Source: CAD feature listing. Evaluate the final solid. Frame: model axes, mm. Give positions to 0.01 mm unless a question says otherwise; leave off trailing zeros. Loops run counter-clockwise (first coordinate to the right, second up) from the corner with the lowest first, then second, coordinate; pieces in that order, holes last. Notation, with made-up numbers: M 80.5,-3.5 L 116.5,-3.5 A27 cw 116.5,31.5 Z; hole C 6.25,32 d10. An arc over 180 degrees is marked long. Put each result on its own line as item: value.
from build123d import *

# Parameters (mm, degrees)
F0_R     = 14.75
F1_DEPTH = 77
F2_R     = 9.55
F3_DEPTH = 77.001
F4_R     = 3


# Not quite as in the source:
# - a fillet or chamfer that OpenCascade refuses, or shapes differently, is made with other operations: its cross-section is extruded or revolved along the edge and cut away or added


with BuildPart() as f1:
    # F0 (on Top) → F1 (new body)
    with BuildSketch(Plane.XY):
        Circle(F0_R)
    extrude(amount=F1_DEPTH)

    # F2 (on Top) → F3 (cut, through all)
    with BuildSketch(Plane.XY):
        Circle(F2_R)
    extrude(amount=F3_DEPTH, mode=Mode.SUBTRACT)

    # F4
    f4_edges = [f1.edges().sort_by_distance(p)[0] for p in [
        (-14.75, 0, 77),
    ]]
    fillet(f4_edges, radius=F4_R)

    # F5: chamfer of 3 on 1 edges, made by hand

    # F5_s1 → F5_t2 (revolve, cut)
    with BuildSketch(Plane.XZ):
        Polygon((12.55, 77), (9.55, 74), (9.55, 77), align=None)
    revolve(axis=Axis((0, 0, 77), (0, 0, -1)), mode=Mode.SUBTRACT)


solid = f1.part
1. Contact query for flat-ended pins moving along their axis: P1, Ø2, axis at y = 1.5, z = 10.5, coming from the +X side; P2, Ø8, axis at y = 7, z = 19.5, coming from the -X side; P3, Ø3, axis at y = -6, z = 49.5, coming from the +X side. Output: stop coordinate, or through.
Found:
P1: x = 14.74
P2: x = -14.44
P3: x = 14.05
2. Section query A-A (x = 0). Output: boundary loops of the cut face in (y, z).
Found:
outline: M -14.75,0 L -9.55,0 L -9.55,74 L -12.46,76.91 A3 ccw -14.75,74 Z; M 9.55,0 L 14.75,0 L 14.75,74 A3 ccw 12.46,76.91 L 9.55,74 Z
3. Material intervals for line 1 (Y direction, x = 0, z = 55); line 2 (X direction, y = 7, z = 70.5); line 3 (X direction, y = 3, z = 32), sorted ascending. Write a range as from..to.
Found:
line 1: -14.75..-9.55, 9.55..14.75
line 2: -12.98..-6.5, 6.5..12.98
line 3: -14.44..-9.07, 9.07..14.44
4. Draft query along X for faces 1 (the cylindrical face through (-7.58, -5.81, 36.48)), 2 (the cylindrical face through (14.07, 4.43, 36.48)), 3 (the flat face through (0, -10, 0)). Return one class per face: pulls with the +X half, pulls with the -X half, needs draft (parallel to the pull), parting line crosses it, or undercut.
Found:
face 1: undercut
face 2: parting line crosses it
face 3: needs draft
5. Section query C-C (z = 70). Output: boundary loops of the cut face in (x, y), plus the area to 3 significant figures.
Found:
outline: C 0,0 d29.5; hole C 0,0 d19.1
area: 397 mm^2
